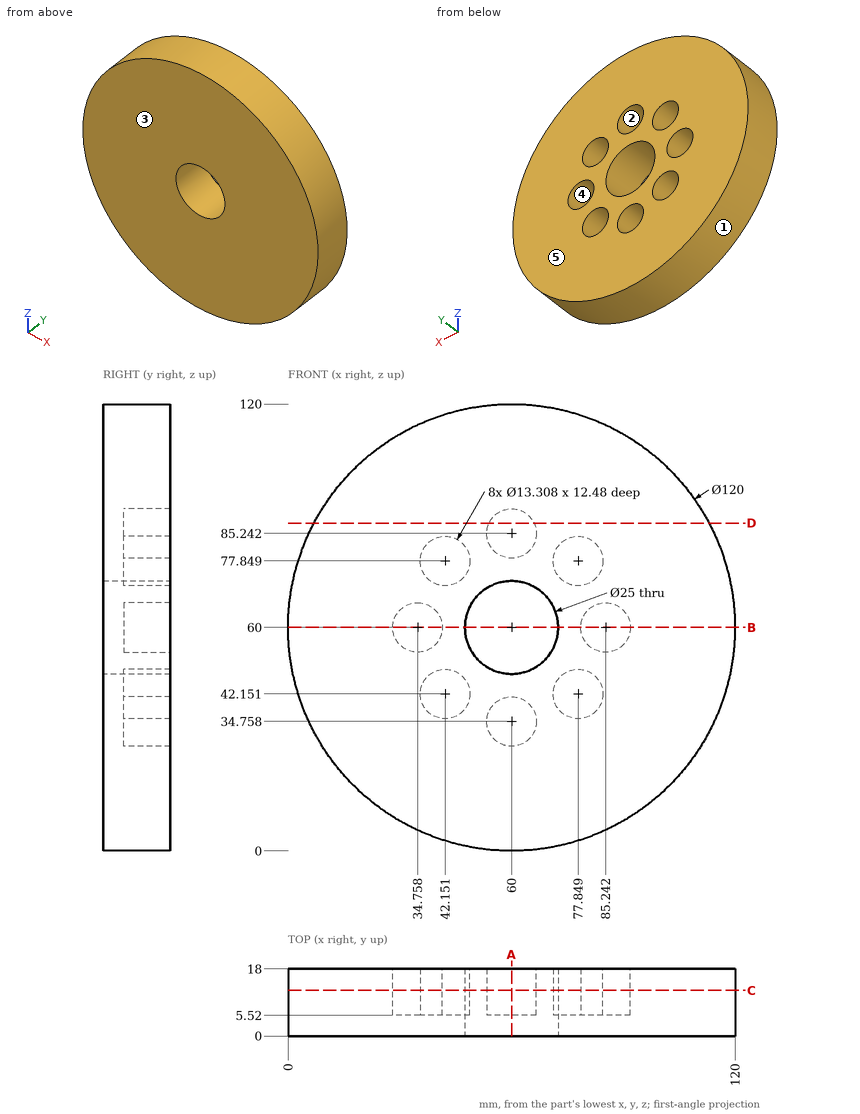
Design review of the part shown in the three views and the two pictorial views. Dimensions are in mm from the part's minimum x, y and z. A direction names the side the tool comes from. Round coordinates to 2 decimals unless told otherwise and drop trailing zeros. Loops run counter-clockwise (first coordinate to the right, second up) from the corner with the lowest first, then second, coordinate; pieces in that order, holes last. Notation, with made-up numbers: M 59,78 L 102,78 A17 cw 102,103 Z; hole C -12,37 d5. An arc over 180 degrees is marked long. Answer as a JSON object with one key per item and string values.
Item 1: We need section A-A, the plane x = 60. State the section outline as (y, z) points.
Check sheet entries:
{"outline": "M 0,0 L 18,0 L 18,28.1 L 5.52,28.1 L 5.52,41.41 L 18,41.41 L 18,47.5 L 0,47.5 Z; M 0,72.5 L 18,72.5 L 18,78.59 L 5.52,78.59 L 5.52,91.9 L 18,91.9 L 18,120 L 0,120 Z"}
Item 2: Tool access review of the marked faces 4 and 5: name each direction out of +Z, -Z, +X, -X, +Y, -Y from which nothing blocks a thin tool from reaching the whole face with its end or side.
Check sheet entries:
{"face 4": "+Y", "face 5": "+Z, -Z, +X, -X, +Y"}
Item 3: We need section B-B, the plane z = 60. State the section outline as (x, y) points.
Check sheet entries:
{"outline": "M 0,0 L 47.5,0 L 47.5,18 L 41.41,18 L 41.41,5.52 L 28.1,5.52 L 28.1,18 L 0,18 Z; M 72.5,0 L 120,0 L 120,18 L 91.9,18 L 91.9,5.52 L 78.59,5.52 L 78.59,18 L 72.5,18 Z"}
Item 4: Clearance check with flat-ended pins moving along their axes: P1, Ø6, axis at y = 9, z = 106, coming from the +X side (1 decimal); P2, Ø12, axis at x = 42.15, z = 77.85, coming from the +Y side; P3, Ø10.5, axis at x = 60, z = 85.24, coming from the -Y side; P4, Ø6, axis at y = 6.5, z = 87.5, coming from the +X side. State where each tip first meets the part, or that it passes through.
Check sheet entries:
{"P1": "x = 101.8", "P2": "y = 5.52", "P3": "y = 0", "P4": "x = 114.77"}
Item 5: We need section D-D, the plane z = 88. State the section outline as (x, y) points.
Check sheet entries:
{"outline": "M 6.93,0 L 113.07,0 L 113.07,18 L 66.06,18 L 66.06,5.52 L 53.94,5.52 L 53.94,18 L 6.93,18 Z"}
Item 6: The part is to be moulded in two halves that separate along Z. For the marked faces 1, 2 and 3, say which applies: +Z half, -Z half, draft (parallel to the pull), parting line (faces both ways), or undercut.
Check sheet entries:
{"face 1": "parting line", "face 2": "undercut", "face 3": "draft"}
Item 7: For line 1 along X through (y, z) = (13, 60); line 2 along X through (y, z) = (15, 38); line 3 along Z through (x, y) = (39, 13) (1 decimal), list the stretches that pass through material, from the lowest coordinate up.
Check sheet entries:
{"line 1": "0 to 28.1, 41.41 to 47.5, 72.5 to 78.59, 91.9 to 120", "line 2": "4.18 to 36.95, 47.35 to 54.19, 65.81 to 72.65, 83.05 to 115.82", "line 3": "3.8 to 36.3, 48 to 54.9, 65.1 to 72, 83.7 to 116.2"}
Item 8: We need section C-C, the plane y = 12.25. State how many separate pieces and enclosed holes the cut face has, and give its area (3 significant figures).
Check sheet entries:
{"separate pieces": "1", "enclosed holes": "9", "area": "9,710 mm2"}
